Autodesk Fusion 360 part; units mm, degrees
sketch "Esquisse1" plane through (0, 0, 0) normal (0, 0, 1) x (1, 0, 0)
  line L0 (0, 0) -> (100, 0)
  line L1 (100, 0) -> (100, 50)
  line L2 (100, 50) -> (0, 50)
  line L3 (0, 50) -> (0, 0)
  dimension "d1" = 100
  dimension "d2" = 50
extrude "Extrusion1" add sketch "Esquisse1" along normal blind 60
sketch "Esquisse2" plane through (0, 0, 0) normal (-1, 0, 0) x (0, -1, 0)
  line L0 (-50, 0) -> (0, 0)
  line L1 (0, 0) -> (0, 60)
  line L2 (0, 60) -> (-50, 60)
  line L3 (-50, 60) -> (-50, 0)
  line L4 (-35, 0) -> (-15, 0)
  line L5 (-15, 0) -> (-15, 40)
  line L6 (-15, 40) -> (-35, 40)
  line L7 (-35, 40) -> (-35, 0)
  dimension "d5" = 15
  dimension "d6" = 20
  dimension "d7" = 40
extrude "Extrusion2" cut 1 faces at (33.3333, 33.3333, 60) along direction (0, 0, -1) blind 10
extrude "Extrusion3" cut sketch "Esquisse2" against normal blind 122 contours L0 L4 L5 L6 L7
extrude "Extrusion4" cut 1 faces at (100, 5, 30) along direction (-1, 0, 0) blind 20
sketch "Esquisse5" plane through (0, 0, 0) normal (-1, 0, 0) x (0, -1, 0)
  line L0 (-15, 40) -> (-15, 0)
  line L1 (-15, 0) -> (0, 0)
  line L2 (0, 0) -> (0, 50)
  line L3 (0, 50) -> (-50, 50)
  line L4 (-50, 50) -> (-50, 0)
  line L5 (-50, 0) -> (-35, 0)
  line L6 (-35, 0) -> (-35, 40)
  line L7 (-35, 40) -> (-15, 40)
  line L8 (-35, 0) -> (-35, 10)
  line L9 (-35, 10) -> (-50, 0)
  line L10 (-15, 0) -> (-15, 10)
  line L11 (-15, 10) -> (0, 0)
  dimension "d14" = 10
  dimension "d15" = 10
extrude "Extrusion5" cut sketch "Esquisse5" against normal blind 285 contours L0 L1 L10 L11 | L5 L6 L8 L9
sketch "Esquisse7" plane through (0, 0, 0) normal (0, -1, 0) x (1, 0, 0)
  line L0 (80, 0) -> (80, 50)
  line L1 (80, 50) -> (0, 50)
  line L2 (0, 50) -> (0, 0)
  line L3 (0, 0) -> (80, 0)
  line L4 (80, 0) -> (65, 0)
  line L5 (65, 0) -> (65, 5)
  line L6 (65, 5) -> (80, 5)
  line L7 (80, 5) -> (80, 0)
  dimension "d18" = 5
  dimension "d19" = 15
extrude "Extrusion6" add sketch "Esquisse7" along normal blind 15 contours L0 L3 L4 L5 L6 L7
sketch "Esquisse9" plane through (0, 0, 5) normal (0, 0, 1) x (-1, 0, 0)
  line L0 (-80, 0) -> (-65, 0)
  line L1 (-65, 0) -> (-65, 15)
  line L2 (-65, 15) -> (-80, 15)
  line L3 (-80, 15) -> (-80, 0)
  line L4 (-65, 0) -> (-80, 15)
  line L5 (-65, 15) -> (-80, 0)
  circle A0 centre (-72.5, 7.5) radius 5
  dimension "d22" = 10
extrude "Extrusion7" cut sketch "Esquisse9" against normal blind 3.5 contours L4 L5 A0 | L4 L5 A0 | L4 L5 A0 | L4 L5 A0
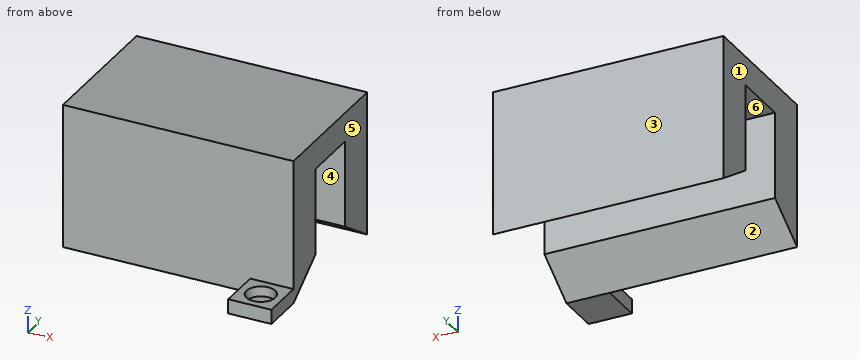
Part model, mm, in its own coordinate system. Face numbers are marked on the shaded views. A direction names the side the tool comes from. Give positions to 0.01 mm unless a question says otherwise; leave off trailing zeros. Order: outer loops, then holes, each group sorted by start corner. A loop starts at its lowest first (then second) coordinate and runs counter-clockwise, first axis right, second up. Notation, with made-up numbers: (3, 83.5) - (26, 83.5) arc R25 cw to (26, 105.5) - close; hole circle Ø7 at (58.5, -8.5). An arc over 180 degrees is marked (long way). Use a Markdown table: item, result.
1) Saw through at B-B on x = 63. List the corners of the cut face in (y, z), plus the area to 3 significant figures.
Checked values:
| item | result |
|---|---|
| outline | (0, 0) - (15, 10) - (15, 40) - (35, 40) - (35, 10) - (50, 0) - (50, 50) - (0, 50) - close |
| area | 1,550 mm² |
2) Saw through at D-D on z = 38.5. List the corners of the cut face in (x, y), plus the area to 3 significant figures.
Checked values:
| item | result |
|---|---|
| outline | (0, 0) - (80, 0) - (80, 15) - (0, 15) - close; (0, 35) - (80, 35) - (80, 50) - (0, 50) - close |
| area | 2,400 mm² |
3) Saw through at A-A on z = 8.5. List the corners of the cut face in (x, y).
Checked values:
| item | result |
|---|---|
| outline | (0, 0) - (80, 0) - (80, 12.75) - (0, 12.75) - close; (0, 37.25) - (80, 37.25) - (80, 50) - (0, 50) - close |
4) Two-plate mould, pull along Y, no slides. Class the marked faces 1, 2, 3 and 4: +Y half, -Y half, draft (parallel to the pull), parting line (faces both ways), or undercut.
Checked values:
| item | result |
|---|---|
| face 1 | draft |
| face 2 | undercut |
| face 3 | +Y half |
| face 4 | undercut |
5) Flat gauge pins, fed straight in: P1, Ø5, axis at x = 9.5, z = 33, coming from the -Y side; P2, Ø1.5, axis at y = -10.5, z = 2.5, coming from the -X side; P3, Ø2, axis at y = 33.5, z = 38.5, coming from the -X side; P4, Ø8, axis at x = 73, y = -9, coming from the +Z side. Where does each tip first touch, or does it go through?
Checked values:
| item | result |
|---|---|
| P1 | y = 0 |
| P2 | x = 65 |
| P3 | through |
| P4 | z = 5 |
6) Probe L1, parallel to Y at x = 75, z = 19; L2, parallel to Y at x = 72.5, z = 3.75 (3 decimals); L3, parallel to X at y = -7.5, z = 3.1. List the from-to ranges inside material, lowest first. Write a range as from..to.
Checked values:
| item | result |
|---|---|
| L1 | 0..15, 35..50 |
| L2 | -15..-12.5, -2.5..5.625, 44.375..50 |
| L3 | 65..67.5, 77.5..80 |
7) 3-axis set-ups, long thin cutter, end or side, ignore diameter. For the marked faces 5 and 6: which of +Z, -Z, +X, -X, +Y, -Y reach the whole face in a straight line?
Checked values:
| item | result |
|---|---|
| face 5 | +Z, -Z, +X, +Y, -Y |
| face 6 | -Z, +X, -X |
8) Saw through at C-C on y = -7.5. List the corners of the cut face in (x, z), plus the area to 3 significant figures.
Checked values:
| item | result |
|---|---|
| outline | (65, 0) - (80, 0) - (80, 5) - (77.5, 5) - (77.5, 1.5) - (67.5, 1.5) - (67.5, 5) - (65, 5) - close |
| area | 40.0 mm² |
